Verification items for the finished model (mm, model axes). A direction names the side the tool comes from. Give positions to 0.01 mm unless a question says otherwise; leave off trailing zeros. Write each loop counter-clockwise with the first axis right and the second up, starting at its lowest first coordinate (ties: lowest second). Pieces come first, ordered by that corner, then holes. Notation, with made-up numbers: (12, -21) - (59, -21) arc R34 ccw to (59, 13) - close; hole circle Ø8 at (6, -7.75). An arc over 180 degrees is marked (long way). Answer as a JSON object with one key per item and string values. Group by question number.
Item 1: Sectioned sample at C-C, the plane y = 0. Record the boundary of the cut face in (x, z), and give its area (3 significant figures).
Item 2: Go/stop test with flat-tipped pins: pin 1 (4 mm diameter, centred on y = 24, z = 4, fed in from +X); pin 2 (5 mm diameter, centred on y = -34, z = 12, fed in from -X); pin 3 (3 mm diameter, centred on y = 29.5, z = 4.5, fed in from +X). Record where each tip stops, or that it passes through.
Item 3: Scan lines: line 1 along Y through (x, z) = (29, 11.5); line 2 along X through (y, z) = (28.5, 8.5); line 3 along X through (y, z) = (0, 13.75). Record each from-to range of solid material in increasing order. Write a range as [from, to].
Item 4: Tool access check on faces 1 (the face through (-1, 46, 8)), 2 (the face through (92.99, 0.82, 8.38)). Record the directions out of +Z, -Z, +X, -X, +Y, -Y that give a thin tool (end or side, any length) a straight path to the whole face; none if there is none.
Item 5: Draft check along Y on faces 3 (the face through (-1, -46, 8)), 4 (the face through (-100.99, -1.01, 8.38)), 5 (the face through (0, 38, 17)), 6 (the face through (-92.99, -0.82, 8.38)). Enter one of: +Y half, -Y half, draft (parallel to the pull), parting line (faces both ways), or undercut.
Item 6: Sectioned sample at A-A, the plane x = 7.5. Record the boundary of the cut face in (y, z), and give its area (3 significant figures).
Item 7: Sectioned sample at B-B, the plane z = 5. Record the boundary of the cut face in (x, y).
Solid Edge part; units mm, degrees
sketch "Sketch1" plane through (0, 0, 0) normal (0, 0, 1) x (1, 0, 0)
  line L0 (-55, -46) -> (55, -46)
  arc A0 (55, 46) -> (55, -46) centre (55, 0) cw
  line L1 (-55, 46) -> (55, 46)
  arc A1 (-55, 46) -> (-55, -46) centre (-55, 0) ccw
  line L2 (-55.5, 37.5) -> (55.5, 37.5)
  arc A2 (55.5, 37.5) -> (55.5, -37.5) centre (55.5, 0) cw
  line L3 (-55.5, -37.5) -> (55.5, -37.5)
  arc A3 (-55.5, 37.5) -> (-55.5, -37.5) centre (-55.5, 0) ccw
  dimension "D1" = 55
  dimension "D2" = 55
extrude "Protrusion1" add sketch "Sketch1" along normal blind 17
Geometry check:
{
 "1": {"outline": "(-101, 0) - (-93, 0) - (-93, 17) - (-101, 17) - close; (93, 0) - (101, 0) - (101, 17) - (93, 17) - close", "area": "272 mm^2"},
 "2": {"pin 1": "x = 95.4", "pin 2": "x = -88.52", "pin 3": "x = 91.5"},
 "3": {"line 1": "[-46, -37.5], [37.5, 46]", "line 2": "[-91.11, -79.87], [79.87, 91.11]", "line 3": "[-101, -93], [93, 101]"},
 "4": {"face 1": "+Z, -Z, +X, -X, +Y", "face 2": "+Z, -Z"},
 "5": {"face 3": "-Y half", "face 4": "parting line", "face 5": "draft", "face 6": "undercut"},
 "6": {"outline": "(-46, 0) - (-37.5, 0) - (-37.5, 17) - (-46, 17) - close; (37.5, 0) - (46, 0) - (46, 17) - (37.5, 17) - close", "area": "289 mm^2"},
 "7": {"outline": "(-55, -46) - (55, -46) arc R46 ccw to (55, 46) - (-55, 46) arc R46 ccw to start; hole (-55.5, -37.5) - (55.5, -37.5) arc R37.5 ccw to (55.5, 37.5) - (-55.5, 37.5) arc R37.5 ccw to start"}
}
